The model under review builds one solid part; all positions refer to its coordinate system, in mm. Round coordinates to 2 decimals unless told otherwise and drop trailing zeros. Order: outer loops, then holes, each group sorted by start corner. A loop starts at its lowest first (then second) coordinate and runs counter-clockwise, first axis right, second up.
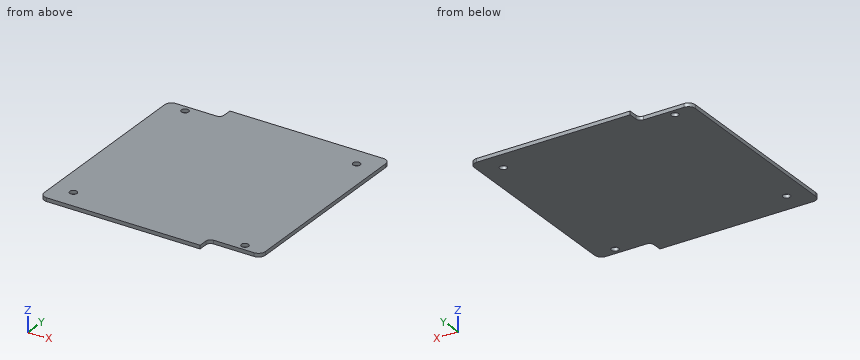
```python
from build123d import *

# Parameters (mm, degrees)
BOSS_EXTRUDE1_DEPTH        = 1.6
F_3_2_3_2_DIAMETER_HOLE3_D = 3.2


with BuildPart() as part:
    # Sketch1 → Boss-Extrude1 (new body)
    with BuildSketch(Plane.XY):
        with BuildLine():
            Line((-16.56534388, -2.04814307), (-84.56534388, -2.04814307))
            ThreePointArc((-84.56534388, -2.04814307), (-86.686664224, -1.169463413), (-87.56534388, 0.95185693))
            Line((-87.56534388, 0.95185693), (-87.56534388, 82.95185693))
            ThreePointArc((-87.56534388, 82.95185693), (-86.686664224, 85.073177274), (-84.56534388, 85.95185693))
            Line((-84.56534388, 85.95185693), (-66.56534388, 85.95185693))
            ThreePointArc((-66.56534388, 85.95185693), (-65.151130318, 86.537643368), (-64.56534388, 87.95185693))
            Line((-64.56534388, 87.95185693), (-64.56534388, 91.95185693))
            Line((-64.56534388, 91.95185693), (3.43465612, 91.95185693))
            ThreePointArc((3.43465612, 91.95185693), (5.555976464, 91.073177274), (6.43465612, 88.95185693))
            Line((6.43465612, 88.95185693), (6.43465612, 6.95185693))
            ThreePointArc((6.43465612, 6.95185693), (5.555976464, 4.830536587), (3.43465612, 3.95185693))
            Line((3.43465612, 3.95185693), (-14.56534388, 3.95185693))
            ThreePointArc((-14.56534388, 3.95185693), (-15.979557442, 3.366070492), (-16.56534388, 1.95185693))
            Line((-16.56534388, 1.95185693), (-16.56534388, -2.04814307))
        make_face()
    extrude(amount=BOSS_EXTRUDE1_DEPTH)

    # Ø3.2 (3.2) Diameter Hole3 (through all)
    with Locations(Plane(origin=(0, 0, 0), x_dir=(-1, 0, 0), z_dir=(0, 0, -1))):
        with Locations((78.56534388, 6.95185693), (78.56534388, 82.95185693), (2.56534388, 82.95185693), (2.56534388, 6.95185693)):
            Hole(F_3_2_3_2_DIAMETER_HOLE3_D / 2)


solid = part.part
```
(1) Consider section B-B (x = -73.5). Write out the cut boundary in (y, z).
Data:
outline: (-2.05, 0) - (85.95, 0) - (85.95, 1.6) - (-2.05, 1.6) - close
(2) To check wall thickness, follow probe 1 along Y at (x, z) = (-80, 0.8); probe 2 along Y at (x, z) = (-4, 1.1); probe 3 along Y at (x, z) = (-8, 1.5). State the ranges of each line that lie inside material, in increasing order.
Data:
probe 1: y = -2.05 to 6.24, 7.66 to 82.24, 83.66 to 85.95
probe 2: y = 3.95 to 6.24, 7.66 to 82.24, 83.66 to 91.95
probe 3: y = 3.95 to 91.95
(3) Consider section A-A (z = 1.2). Write out the cut boundary in (x, y), and give its area (3 significant figures).
Data:
outline: (-87.57, 0.95) arc R3 ccw to (-84.57, -2.05) - (-16.57, -2.05) - (-16.57, 1.95) arc R2 cw to (-14.57, 3.95) - (3.43, 3.95) arc R3 ccw to (6.43, 6.95) - (6.43, 88.95) arc R3 ccw to (3.43, 91.95) - (-64.57, 91.95) - (-64.57, 87.95) arc R2 cw to (-66.57, 85.95) - (-84.57, 85.95) arc R3 ccw to (-87.57, 82.95) - close; hole circle Ø3.2 at (-78.57, 6.95); hole circle Ø3.2 at (-78.57, 82.95); hole circle Ø3.2 at (-2.57, 6.95); hole circle Ø3.2 at (-2.57, 82.95)
area: 8,520 mm2
(4) Insertion check: pin 1 (0.8 mm diameter, centred on x = -8.5, z = 1, fed in from -Y); pin 2 (0.8 mm diameter, centred on y = 0, z = 1, fed in from +X); pin 3 (2.5 mm diameter, centred on x = -78.57, y = 82.95, fed in from -Z) (3 decimals). Each pin has a flat end and moves straight along its axis. Give the tip position at first contact, or say it passes through.
Data:
pin 1: stops at y = 3.95
pin 2: stops at x = -16.57
pin 3: passes through
